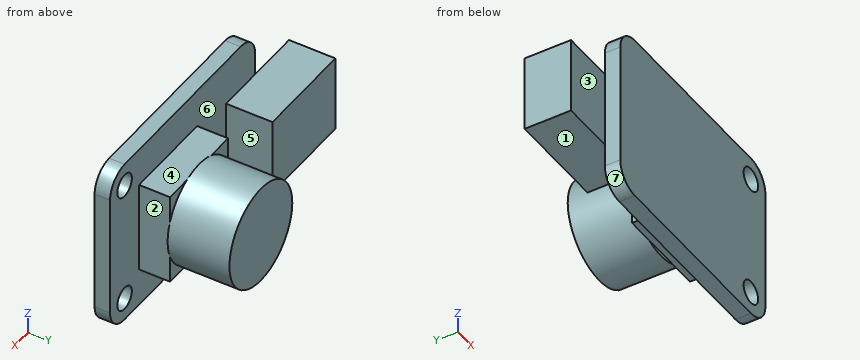
from build123d import *

# Parameters (mm, degrees)
SKETCH1_R           = 1.5
BOSS_EXTRUDE1_DEPTH = 2
SKETCH2_W           = 13
SKETCH2_H           = 10
BOSS_EXTRUDE2_DEPTH = 6
SKETCH4_W           = 12
SKETCH4_H           = 12
BOSS_EXTRUDE4_DEPTH = 4
SKETCH5_R           = 6.5
BOSS_EXTRUDE5_DEPTH = 8


with BuildPart() as part:
    # Sketch1 → Boss-Extrude1 (new body)
    with BuildSketch(Plane(origin=(0, 0, 0), x_dir=(1, 0, 0), z_dir=(0, 1, 0))):
        with BuildLine():
            Line((-12, 11), (12, 11))
            ThreePointArc((12, 11), (14.121320344, 10.121320344), (15, 8))
            Line((15, 8), (15, -8))
            ThreePointArc((15, -8), (14.121320344, -10.121320344), (12, -11))
            Line((12, -11), (-12, -11))
            ThreePointArc((-12, -11), (-14.121320344, -10.121320344), (-15, -8))
            Line((-15, -8), (-15, 8))
            ThreePointArc((-15, 8), (-14.121320344, 10.121320344), (-12, 11))
        make_face()
        with Locations(Location((12, 8, 0), (0, 0, 270))):
            Circle(SKETCH1_R, mode=Mode.SUBTRACT)
        with Locations(Location((12, -8, 0), (0, 0, 270))):
            Circle(SKETCH1_R, mode=Mode.SUBTRACT)
    extrude(amount=BOSS_EXTRUDE1_DEPTH)

    # Sketch2 → Boss-Extrude2 (add)
    with BuildSketch(Plane(origin=(0, 2, 0), x_dir=(1, 0, 0), z_dir=(0, 1, 0))):
        with Locations((-15.5, 0)):
            Rectangle(SKETCH2_W, SKETCH2_H)
    extrude(amount=BOSS_EXTRUDE2_DEPTH)

    # Sketch4 → Boss-Extrude4 (add)
    with BuildSketch(Plane(origin=(0, 2, 0), x_dir=(1, 0, 0), z_dir=(0, 1, 0))):
        with Locations((3, 0)):
            Rectangle(SKETCH4_W, SKETCH4_H)
    extrude(amount=BOSS_EXTRUDE4_DEPTH)

    # Sketch5 → Boss-Extrude5 (add)
    with BuildSketch(Plane(origin=(0, 6, 0), x_dir=(1, 0, 0), z_dir=(0, 1, 0))):
        with Locations(Location((3, 0, 0), (0, 0, 67.380135052))):
            Circle(SKETCH5_R)
    extrude(amount=BOSS_EXTRUDE5_DEPTH)


solid = part.part
Work out the finished part from the listing and answer in its coordinate system (mm). Face numbers are marked on the shaded views. A direction names the side the tool comes from. Coordinates: 2 decimals unless noted, no trailing zeros. Loops run counter-clockwise (first coordinate to the right, second up) from the corner with the lowest first, then second, coordinate; pieces in that order, holes last. Notation, with made-up numbers: (-34, 17) -> (-13, 17) arc R7 cw to (-13, 27) -> close; hole circle Ø6 at (43.25, 26). An arc over 180 degrees is marked (long way). Answer as CSV lines item,"result".
1) For a pull along X with two mould halves and no side action, classify the marked faces 4, 5, 6 and 7 as released by +X, released by -X, zero draft, split by the parting line, or undercut.
A:
face 4,"zero draft"
face 5,"undercut"
face 6,"undercut"
face 7,"released by -X"
2) Straight lines are drawn through the part: probe 1 along X at (y, z) = (1.1, -8); probe 2 along X at (y, z) = (2.5, 0); probe 3 along Y at (x, z) = (2.5, -7). For each, find the intervals that lie inside material, in ascending order.
A:
probe 1,"x = -15 to 10.5, 13.5 to 15"
probe 2,"x = -22 to -9, -3 to 9"
probe 3,"y = 0 to 2"
3) The part is cut by section A-A (y = 7). Give the vertices of the cut face in (x, z).
A:
outline,"(-22, -5) -> (-9, -5) -> (-9, 5) -> (-22, 5) -> close; circle Ø13 at (3, 0)"
4) Flat-ended cylindrical pins translate along their axes: pin 1 (1.2 mm diameter, centred on y = 3.5, z = 1.5, fed in from +X); pin 2 (3.5 mm diameter, centred on x = -20, z = 1, fed in from -Y); pin 3 (6 mm diameter, centred on x = -3.5, y = 5.5, fed in from +Z). Find the tip coordinate at first contact, or state that the pin passes through.
A:
pin 1,"stops at x = 9"
pin 2,"stops at y = 2"
pin 3,"stops at z = 6"
5) The part is cut by section C-C (x = 3). Give the vertices of the cut face in (y, z).
A:
outline,"(0, -11) -> (2, -11) -> (2, -6) -> (6, -6) -> (6, -6.5) -> (14, -6.5) -> (14, 6.5) -> (6, 6.5) -> (6, 6) -> (2, 6) -> (2, 11) -> (0, 11) -> close"
6) For the marked faces 1, 2 and 3, determine the directions among +Z, -Z, +X, -X, +Y, -Y from which every point of the face is accessible in a straight line to the end or side of a thin tool.
A:
face 1,"-Z, -X, +Y"
face 2,"+Z, -Z, +X"
face 3,"+Z, -Z, -X, -Y"
7) The part is cut by section B-B (z = 0). Give the vertices of the cut face in (x, y).
A:
outline,"(-22, 2) -> (-15, 2) -> (-15, 0) -> (15, 0) -> (15, 2) -> (9, 2) -> (9, 6) -> (9.5, 6) -> (9.5, 14) -> (-3.5, 14) -> (-3.5, 6) -> (-3, 6) -> (-3, 2) -> (-9, 2) -> (-9, 8) -> (-22, 8) -> close"
8) The part is cut by section D-D (y = 3.25). Give the vertices of the cut face in (x, z).
A:
outline,"(-22, -5) -> (-9, -5) -> (-9, 5) -> (-22, 5) -> close; (-3, -6) -> (9, -6) -> (9, 6) -> (-3, 6) -> close"
